Part model, mm, in its own coordinate system. A direction names the side the tool comes from. Give positions to 0.01 mm unless a question says otherwise; leave off trailing zeros. Write each loop counter-clockwise with the first axis right and the second up, starting at its lowest first coordinate (ties: lowest second). Pieces come first, ordered by that corner, then holes.
from build123d import *

# Parameters (mm, degrees)
SKETCH_1_W                = 95.5
SKETCH_1_H                = 95.5
SKETCH_1_R                = 9.5
EXTRUDE_1_DEPTH           = 3
SKETCH_3_W                = 42
SKETCH_3_H                = 42
CUT_EXTRUDE_2_DEPTH       = 68.595303091
SKETCH_5_W                = 95.5
SKETCH_5_H                = 95.5
SKETCH_5_W_2              = 89.5
SKETCH_5_H_2              = 89.5
EXTRUDE_2_DEPTH           = 8.3
FILLET_1_R                = 5
SKETCH_7_W                = 48
SKETCH_7_H                = 48
SKETCH_7_W_2              = 42
SKETCH_7_H_2              = 42
EXTRUDE_4_DEPTH           = 8.3
CHAMFER_3_SIZE            = 1.5
CHAMFER_5_SIZE            = 1.5
SKETCH_12_R               = 1.6
CUT_EXTRUDE_8_DEPTH       = 69.467620084
SKETCH_13_W               = 20.75
SKETCH_13_H               = 7
SKETCH_13_W_2             = 7
SKETCH_13_H_2             = 20.75
EXTRUDE_5_DEPTH           = 8.3
SKETCH_14_R               = 1.6
CUT_EXTRUDE_9_DEPTH       = 69.467620084
EXTRUDE_6_REACH           = 70.468
SKETCH_15_W               = 32
SKETCH_15_H               = 1.5
SKETCH_15_W_2             = 1.5
SKETCH_15_H_2             = 32
CUT_EXTRUDE_10_DEPTH      = 69.036865007
CUT_EXTRUDE_10_DEPTH_BACK = 69.036865007
SKETCH_16_W               = 12
SKETCH_16_H               = 12
SKETCH_17_W               = 42
SKETCH_17_H               = 42
EXTRUDE_7_DEPTH           = 11.3
FILLET_2_R                = 2
SKETCH_18_W               = 41.3
SKETCH_18_H               = 41.3
CUT_EXTRUDE_11_DEPTH      = 69.467620084
FILLET_3_R                = 5


with BuildPart() as part:
    # ｽｹｯﾁ1 → ﾎﾞｽ - 押し出し1 (new body)
    with BuildSketch(Plane.XY):
        Rectangle(SKETCH_1_W, SKETCH_1_H)
        with Locations((-34.25, 34.25)):
            Circle(SKETCH_1_R, mode=Mode.SUBTRACT)
        with Locations((34.25, 34.25)):
            Circle(SKETCH_1_R, mode=Mode.SUBTRACT)
        with Locations((34.25, -34.25)):
            Circle(SKETCH_1_R, mode=Mode.SUBTRACT)
        with Locations((-34.25, -34.25)):
            Circle(SKETCH_1_R, mode=Mode.SUBTRACT)
    extrude(amount=EXTRUDE_1_DEPTH)

    # ｽｹｯﾁ3 → ｶｯﾄ - 押し出し2 (cut, through all)
    with BuildSketch(Plane.XY.offset(3)):
        Rectangle(SKETCH_3_W, SKETCH_3_H)
    extrude(amount=-CUT_EXTRUDE_2_DEPTH, mode=Mode.SUBTRACT)

    # ｽｹｯﾁ5 → ﾎﾞｽ - 押し出し2 (add)
    with BuildSketch(Plane.XY.offset(3)):
        Rectangle(SKETCH_5_W, SKETCH_5_H)
        Rectangle(SKETCH_5_W_2, SKETCH_5_H_2, mode=Mode.SUBTRACT)
    extrude(amount=EXTRUDE_2_DEPTH)

    # ﾌｨﾚｯﾄ1
    fillet_1_edges = [part.edges().sort_by_distance(p)[0] for p in [
        (-47.75, 47.75, 5.65),
        (47.75, 47.75, 5.65),
        (47.75, -47.75, 5.65),
        (-47.75, -47.75, 5.65),
    ]]
    fillet(fillet_1_edges, radius=FILLET_1_R)

    # ｽｹｯﾁ7 → ﾎﾞｽ - 押し出し4 (add)
    with BuildSketch(Plane.XY.offset(3)):
        Rectangle(SKETCH_7_W, SKETCH_7_H)
        Rectangle(SKETCH_7_W_2, SKETCH_7_H_2, mode=Mode.SUBTRACT)
    extrude(amount=EXTRUDE_4_DEPTH)

    # 面取り3
    chamfer_3_edges = [part.edges().sort_by_distance(p)[0] for p in [
        (47.75, 0, 0),
        (-47.75, 0, 0),
        (0, 47.75, 0),
        (0, -47.75, 0),
        (-46.285533906, 46.285533906, 0),
        (46.285533906, 46.285533906, 0),
        (-46.285533906, -46.285533906, 0),
        (46.285533906, -46.285533906, 0),
    ]]
    chamfer(chamfer_3_edges, length=CHAMFER_3_SIZE)

    # 面取り5
    chamfer_5_edges = [part.edges().sort_by_distance(p)[0] for p in [
        (-43.75, 34.25, 0),
        (24.75, 34.25, 0),
        (24.75, -34.25, 0),
        (-43.75, -34.25, 0),
    ]]
    chamfer(chamfer_5_edges, length=CHAMFER_5_SIZE)

    # ｽｹｯﾁ12 → ｶｯﾄ - 押し出し8 (cut, through all)
    with BuildSketch(Plane(origin=(0, 0, 0), x_dir=(-1, 0, 0), z_dir=(0, 0, -1))):
        with Locations((-0.15, 39.15)):
            Circle(SKETCH_12_R)
        with Locations((-39.15, -0.15)):
            Circle(SKETCH_12_R)
        with Locations((39.15, 0.15)):
            Circle(SKETCH_12_R)
        with Locations((0.15, -39.15)):
            Circle(SKETCH_12_R)
    extrude(amount=-CUT_EXTRUDE_8_DEPTH, mode=Mode.SUBTRACT)

    # ｽｹｯﾁ13 → ﾎﾞｽ - 押し出し5 (add)
    with BuildSketch(Plane.XY.offset(3)):
        with Locations((-34.375, -0.25)):
            Rectangle(SKETCH_13_W, SKETCH_13_H)
        with Locations((0.25, -34.375)):
            Rectangle(SKETCH_13_W_2, SKETCH_13_H_2)
        with Locations((34.375, 0.25)):
            Rectangle(SKETCH_13_W, SKETCH_13_H)
        with Locations((-0.25, 34.375)):
            Rectangle(SKETCH_13_W_2, SKETCH_13_H_2)
    extrude(amount=EXTRUDE_5_DEPTH)

    # ｽｹｯﾁ14 → ｶｯﾄ - 押し出し9 (cut, through all)
    with BuildSketch(Plane.XY.offset(11.3)):
        with Locations(Location((-39.15, 0.15, 0), (0, 0, 180))):
            Circle(SKETCH_14_R)
        with Locations(Location((-0.15, -39.15, 0), (0, 0, 180))):
            Circle(SKETCH_14_R)
        with Locations(Location((39.15, -0.15, 0), (0, 0, 180))):
            Circle(SKETCH_14_R)
        with Locations(Location((0.15, 39.15, 0), (0, 0, 180))):
            Circle(SKETCH_14_R)
    extrude(amount=-CUT_EXTRUDE_9_DEPTH, mode=Mode.SUBTRACT)

    # ﾎﾞｽ - 押し出し6: up to this face of the body (flat: up to its plane)
    extrude_6_end = Plane(part.part.faces().sort_by_distance((0, -46.399426048, 11.3))[0])
    # ｽｹｯﾁ15 → ﾎﾞｽ - 押し出し6 (add, up to the picked face)
    with BuildSketch(Plane(origin=(0, 0, 0), x_dir=(-1, 0, 0), z_dir=(0, 0, -1)), mode=Mode.PRIVATE) as extrude_6_sk1:
        with Locations((0, 47)):
            Rectangle(SKETCH_15_W, SKETCH_15_H)
    extrude_6_tool1 = split(extrude(extrude_6_sk1.sketch, amount=-EXTRUDE_6_REACH, mode=Mode.PRIVATE), bisect_by=extrude_6_end, keep=Keep.BOTH, mode=Mode.PRIVATE)
    # ｽｹｯﾁ15 → ﾎﾞｽ - 押し出し6 (add, up to the picked face)
    with BuildSketch(Plane(origin=(0, 0, 0), x_dir=(-1, 0, 0), z_dir=(0, 0, -1)), mode=Mode.PRIVATE) as extrude_6_sk2:
        with Locations((47, 0)):
            Rectangle(SKETCH_15_W_2, SKETCH_15_H_2)
    extrude_6_tool2 = split(extrude(extrude_6_sk2.sketch, amount=-EXTRUDE_6_REACH, mode=Mode.PRIVATE), bisect_by=extrude_6_end, keep=Keep.BOTH, mode=Mode.PRIVATE)
    # ｽｹｯﾁ15 → ﾎﾞｽ - 押し出し6 (add, up to the picked face)
    with BuildSketch(Plane(origin=(0, 0, 0), x_dir=(-1, 0, 0), z_dir=(0, 0, -1)), mode=Mode.PRIVATE) as extrude_6_sk3:
        with Locations((0, -47)):
            Rectangle(SKETCH_15_W, SKETCH_15_H)
    extrude_6_tool3 = split(extrude(extrude_6_sk3.sketch, amount=-EXTRUDE_6_REACH, mode=Mode.PRIVATE), bisect_by=extrude_6_end, keep=Keep.BOTH, mode=Mode.PRIVATE)
    # ｽｹｯﾁ15 → ﾎﾞｽ - 押し出し6 (add, up to the picked face)
    with BuildSketch(Plane(origin=(0, 0, 0), x_dir=(-1, 0, 0), z_dir=(0, 0, -1)), mode=Mode.PRIVATE) as extrude_6_sk4:
        with Locations((-47, 0)):
            Rectangle(SKETCH_15_W_2, SKETCH_15_H_2)
    extrude_6_tool4 = split(extrude(extrude_6_sk4.sketch, amount=-EXTRUDE_6_REACH, mode=Mode.PRIVATE), bisect_by=extrude_6_end, keep=Keep.BOTH, mode=Mode.PRIVATE)
    add(extrude_6_tool1.solids().sort_by(Axis((0, 47, 0), (0, 0, 1)))[0])
    add(extrude_6_tool2.solids().sort_by(Axis((-47, 0, 0), (0, 0, 1)))[0])
    add(extrude_6_tool3.solids().sort_by(Axis((0, -47, 0), (0, 0, 1)))[0])
    add(extrude_6_tool4.solids().sort_by(Axis((47, 0, 0), (0, 0, 1)))[0])

    # ｽｹｯﾁ16 → ｶｯﾄ - 押し出し10 (cut, two sides: drawn at the far end of the back side and taken through both)
    with BuildSketch(Plane.XY.offset(3).offset(-CUT_EXTRUDE_10_DEPTH_BACK)):
        with Locations((9.25, 29.75)):
            Rectangle(SKETCH_16_W, SKETCH_16_H)
        with Locations((29.75, -9.25)):
            Rectangle(SKETCH_16_W, SKETCH_16_H)
        with Locations((-9.25, -29.75)):
            Rectangle(SKETCH_16_W, SKETCH_16_H)
        with Locations((-29.75, 9.25)):
            Rectangle(SKETCH_16_W, SKETCH_16_H)
    extrude(amount=CUT_EXTRUDE_10_DEPTH + CUT_EXTRUDE_10_DEPTH_BACK, mode=Mode.SUBTRACT)

    # ｽｹｯﾁ17 → ﾎﾞｽ - 押し出し7 (add, through all)
    with BuildSketch(Plane(origin=(0, 0, 0), x_dir=(-1, 0, 0), z_dir=(0, 0, -1))):
        Rectangle(SKETCH_17_W, SKETCH_17_H)
    extrude(amount=-EXTRUDE_7_DEPTH)

    # ﾌｨﾚｯﾄ2
    fillet_2_edges = [part.edges().sort_by_distance(p)[0] for p in [
        (3.25, 35.75, 1.5),
        (15.25, 35.75, 1.5),
        (15.25, 23.75, 5.65),
        (3.25, 23.75, 5.65),
        (-35.75, 15.25, 1.5),
        (-35.75, 3.25, 1.5),
        (-23.75, 3.25, 5.65),
        (-23.75, 15.25, 5.65),
        (-15.25, -23.75, 5.65),
        (-3.25, -23.75, 5.65),
        (-3.25, -35.75, 1.5),
        (-15.25, -35.75, 1.5),
        (23.75, -15.25, 5.65),
        (35.75, -15.25, 1.5),
        (35.75, -3.25, 1.5),
        (23.75, -3.25, 5.65),
    ]]
    fillet(fillet_2_edges, radius=FILLET_2_R)

    # ｽｹｯﾁ18 → ｶｯﾄ - 押し出し11 (cut, through all)
    with BuildSketch(Plane(origin=(0, 0, 0), x_dir=(-1, 0, 0), z_dir=(0, 0, -1))):
        Rectangle(SKETCH_18_W, SKETCH_18_H)
    extrude(amount=-CUT_EXTRUDE_11_DEPTH, mode=Mode.SUBTRACT)

    # ﾌｨﾚｯﾄ3
    fillet_3_edges = [part.edges().sort_by_distance(p)[0] for p in [
        (-20.65, 20.65, 5.65),
        (-20.65, -20.65, 5.65),
        (20.65, -20.65, 5.65),
        (20.65, 20.65, 5.65),
    ]]
    fillet(fillet_3_edges, radius=FILLET_3_R)


solid = part.part
1) 3-axis set-ups, long thin cutter, end or side, ignore diameter. For faces 1 (the flat face through (-23.75, 9, 6)), 2 (the cylindrical face through (-46.32, -46.25, 6.47)), 3 (the flat face through (14, -24, 7)): which of +Z, -Z, +X, -X, +Y, -Y reach the whole face in a straight line?
Check result:
face 1: +Z, -Z
face 2: +Z, -Z, -X, -Y
face 3: +Z
2) Saw through at C-C (z = 6.75). State how many separate pieces and enclosed holes the cut face has, and give its area (3 significant figures).
Check result:
separate pieces: 1
enclosed holes: 9
area: 2,250 mm2
3) Drill centre lines: L1, parallel to Y at x = 39.15, z = 7.75; L2, parallel to Y at x = -23.5, z = 4; L3, parallel to X at y = 39.15, z = 4.5. Where is each one in solid material? Low to high.
Check result:
L1: y = -47.75 to -44.75, -3.25 to -1.75, 1.45 to 3.75, 44.75 to 47.75
L2: y = -47.75 to -44.75, -24 to 24, 44.75 to 47.75
L3: x = -47.75 to -44.75, -3.75 to -1.45, 1.75 to 3.25, 44.75 to 47.75
4) Mould opens along Y. For faces 4 (the cylindrical face through (46.25, -46.32, 6.47)), 5 (the cylindrical face through (46.32, 46.25, 6.33)), 6 (the flat face through (-35, 3.25, 6)) say: +Y half, -Y half, draft (parallel to the pull), parting line (faces both ways), or undercut.
Check result:
face 4: -Y half
face 5: +Y half
face 6: undercut
5) Saw through at B-B (x = 0.15). Write the cut outline in (y, z), and give its area (3 significant figures).
Check result:
outline: (-47.75, 0) - (-40.72, 0) - (-40.72, 11.3) - (-47.75, 11.3) - close; (-37.58, 0) - (-20.65, 0) - (-20.65, 11.3) - (-37.58, 11.3) - close; (20.65, 0) - (37.55, 0) - (37.55, 11.3) - (20.65, 11.3) - close; (40.75, 0) - (47.75, 0) - (47.75, 11.3) - (40.75, 11.3) - close
area: 541 mm2
6) Saw through at A-A (y = -17.5). Write the cut outline in (x, z).
Check result:
outline: (-47.75, 1.5) - (-46.25, 0) - (-20.3, 0) - (-20.3, 11.3) - (-24, 11.3) - (-24, 3) - (-44.75, 3) - (-44.75, 11.3) - (-47.75, 11.3) - close; (20.3, 0) - (46.25, 0) - (47.75, 1.5) - (47.75, 11.3) - (44.75, 11.3) - (44.75, 3) - (24, 3) - (24, 11.3) - (20.3, 11.3) - close
7) Flat gauge pins, fed straight in: P1, Ø15, axis at x = 34.25, y = -34.25, coming from the +Z side; P2, Ø2, axis at x = 34, y = -19.5, coming from the +Z side. Where does each tip first touch, or does it go through?
Check result:
P1: passes through
P2: stops at z = 3
